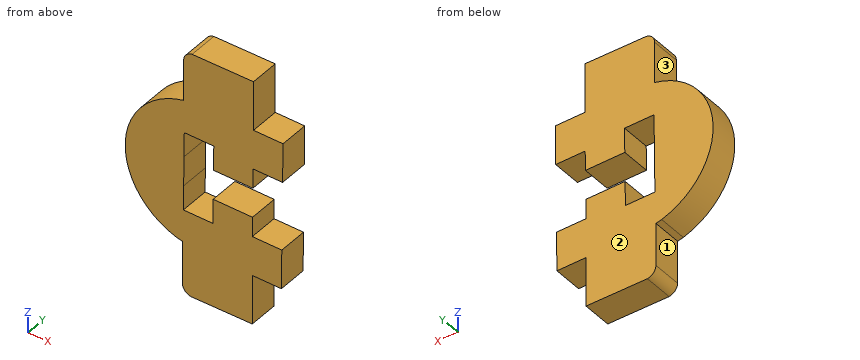
from build123d import *

# Parameters (mm, degrees)
SALIENTE_EXTRUIR1_DEPTH = 3


with BuildPart() as part:
    # Croquis1 → Saliente-Extruir1 (new body)
    with BuildSketch(Plane(origin=(0, 0, 0), x_dir=(1, 0, 0), z_dir=(0, 1, 0))):
        with BuildLine():
            Line((33638.899606001, 12674.802256187), (33638.31321683, 12674.669512098))
            ThreePointArc((33638.31321683, 12674.669512098), (33633.089099042, 12667.180361564), (33639.024595085, 12660.24143736))
            Line((33639.024595085, 12660.24143736), (33639.024595085, 12656.099650441))
            ThreePointArc((33639.024595085, 12656.099650441), (33639.269455485, 12655.444618543), (33639.883952447, 12655.11082686))
            Line((33639.883952447, 12655.11082686), (33646.127320324, 12655.11082686))
            Line((33646.127320324, 12655.11082686), (33646.127126628, 12660.11082686))
            Line((33646.127126628, 12660.11082686), (33649.127126628, 12660.144916986))
            Line((33649.127126628, 12660.144916986), (33649.081676061, 12664.144658758))
            Line((33649.081676061, 12664.144658758), (33646.081869732, 12664.110570833))
            Line((33646.081869732, 12664.110570833), (33646.059144449, 12666.11044172))
            Line((33646.059144449, 12666.11044172), (33642.059402676, 12666.064991153))
            Line((33642.059402676, 12666.064991153), (33642.087809281, 12663.565152545))
            Line((33642.087809281, 12663.565152545), (33639.088002951, 12663.53106462))
            Line((33639.088002951, 12663.53106462), (33639.059596347, 12666.030903228))
            Line((33639.059596347, 12666.030903228), (33639.025508422, 12669.030709557))
            Line((33639.025508422, 12669.030709557), (33638.997101818, 12671.530548165))
            Line((33638.997101818, 12671.530548165), (33641.996908147, 12671.56463609))
            Line((33641.996908147, 12671.56463609), (33642.025314751, 12669.064797482))
            Line((33642.025314751, 12669.064797482), (33646.025056524, 12669.110248049))
            Line((33646.025056524, 12669.110248049), (33646.00233124, 12671.110118935))
            Line((33646.00233124, 12671.110118935), (33649.00213757, 12671.14420686))
            Line((33649.00213757, 12671.14420686), (33648.956687003, 12675.143948633))
            Line((33648.956687003, 12675.143948633), (33646.00233124, 12675.110377179))
            Line((33646.00233124, 12675.110377179), (33646.00233124, 12680.110377179))
            Line((33646.00233124, 12680.110377179), (33639.758963363, 12680.110377179))
            ThreePointArc((33639.758963363, 12680.110377179), (33639.144466402, 12679.776585497), (33638.899606001, 12679.121553599))
            Line((33638.899606001, 12679.121553599), (33638.899606001, 12674.802256187))
        make_face()
    extrude(amount=SALIENTE_EXTRUIR1_DEPTH)


solid = part.part
Source: CAD feature listing. Evaluate the final solid. Frame: model axes, mm. Face numbers are marked on the shaded views. A direction names the side the tool comes from. Round coordinates to 2 decimals unless told otherwise and drop trailing zeros. Write each loop counter-clockwise with the first axis right and the second up, starting at its lowest first coordinate (ties: lowest second). Pieces come first, ordered by that corner, then holes. Notation, with made-up numbers: M 26,27.25 L 75,27.25 A8 ccw 75,34.25 Z; hole C 65.25,59 d11. An arc over 180 degrees is marked long. One line per item, written item: value. Start each with the question number.
Item 1: Ray query, L1, parallel to Z at x = 33641, y = 0.4; L2, parallel to X at y = 2.85, z = -12671; L3, parallel to Z at x = 33645, y = 1. Return the intervals inside material, ascending. Write a range as from..to.
Item 2: Section query C-C (y = 1.2). Return the cut outline in (x, z) (1 decimal), plus the area to 3 significant figures.
Item 3: Set-up query: the marked faces 1, 2 and 3. Return all of +Z, -Z, +X, -X, +Y, -Y with unobstructed straight access to the full face (end or side cutting, diameter ignored); none if empty.
Item 4: Section query D-D (z = -12678). Return the cut outline in (x, y).
Item 5: Section query A-A (z = -12670.5). Return the cut outline in (x, y).
Item 6: Section query B-B (x = 33643.25). Return the cut outline in (y, z), plus the area to 3 significant figures.
Item 7: Pin query (flat end, axial travel): pin 1 (0.9 mm diameter, centred on y = 2, z = -12657, fed in from -X); pin 2 (0.9 mm diameter, centred on y = 1.5, z = -12658, fed in from +X); pin 3 (0.9 mm diameter, centred on y = 1.5, z = -12677.5, fed in from +X). Return the tip coordinate at first contact, or that it passes through.
Result set:
1. L1: z = -12680.11..-12671.55, -12663.55..-12655.11
1. L2: x = 33633.93..33639, 33642..33646
1. L3: z = -12680.11..-12669.1, -12666.1..-12655.11
2. outline: M 33638.3,-12674.7 L 33638.9,-12674.8 L 33638.9,-12679.1 A1 ccw 33639.8,-12680.1 L 33646,-12680.1 L 33646,-12675.1 L 33649,-12675.1 L 33649,-12671.1 L 33646,-12671.1 L 33646,-12669.1 L 33642,-12669.1 L 33642,-12671.6 L 33639,-12671.5 L 33639.1,-12663.5 L 33642.1,-12663.6 L 33642.1,-12666.1 L 33646.1,-12666.1 L 33646.1,-12664.1 L 33649.1,-12664.1 L 33649.1,-12660.1 L 33646.1,-12660.1 L 33646.1,-12655.1 L 33639.9,-12655.1 A1 ccw 33639,-12656.1 L 33639,-12660.2 A7.5 ccw Z
2. area: 229 mm²
3. face 1: -Z, -X, +Y, -Y
3. face 2: +Z, -Z, +X, -X, +Y
3. face 3: +Z, -X, +Y, -Y
4. outline: M 33638.9,0 L 33646,0 L 33646,3 L 33638.9,3 Z
5. outline: M 33633.69,0 L 33639.01,0 L 33639.01,3 L 33633.69,3 Z; M 33642.01,0 L 33646.01,0 L 33646.01,3 L 33642.01,3 Z
6. outline: M 0,-12680.11 L 3,-12680.11 L 3,-12669.08 L 0,-12669.08 Z; M 0,-12666.08 L 3,-12666.08 L 3,-12655.11 L 0,-12655.11 Z
6. area: 66.0 mm²
7. pin 1: stops at x = 33639.02
7. pin 2: stops at x = 33646.13
7. pin 3: stops at x = 33646
